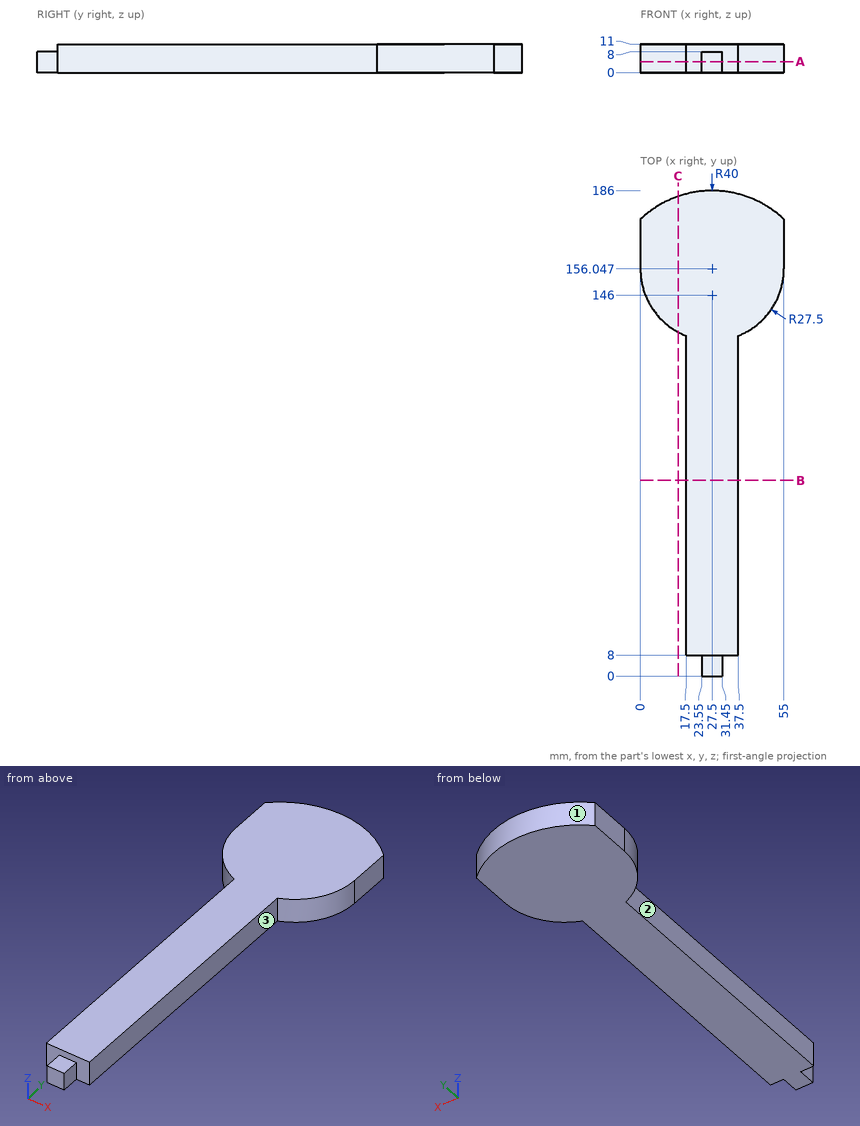
Input: dimensioned drawing with shaded views. Units: mm. Origin: part minimum x, y, z. A direction names the side the tool comes from. Give positions to 0.01 mm unless a question says otherwise; leave off trailing zeros. Loops run counter-clockwise (first coordinate to the right, second up) from the corner with the lowest first, then second, coordinate; pieces in that order, holes last. Notation, with made-up numbers: M -12.75,1 L 29.25,1 A12 ccw 29.25,10 Z; hole C 33,25.5 d2. An arc over 180 degrees is marked long. Put each result on its own line as item: value. Start each with the question number.
1) Access query for the marked faces 1, 2 and 3. Directions: +Z, -Z, +X, -X, +Y, -Y. A direction counts if a zero-diameter tool reaches every point of the face in a straight line with its end or side. Return the directions, or none.
2) Ray query, line 1 along X through (y, z) = (45.5, 10.75); line 2 along Y through (x, z) = (27, 2.75); line 3 along Y through (x, z) = (40, 6.75). Return the intervals inside material, ascending.
3) Cut plane A-A (z = 4.25). Output: boundary loops of the cut face in (x, y), then the cut area to 3 significant figures.
4) Contact query for flat-ended pins moving along their axis: pin 1 (2 mm diameter, centred on y = 54.5, z = 5, fed in from -X); pin 2 (2 mm diameter, centred on x = 10, z = 5.5, fed in from -Y); pin 3 (2 mm diameter, centred on x = 40, z = 3, fed in from -Y). Output: stop coordinate, or through.
5) Cut plane C-C (x = 14.5). Output: boundary loops of the cut face in (y, z) (1 decimal), then the cut area to 3 significant figures.
6) Cut plane B-B (y = 75). Output: boundary loops of the cut face in (x, z).
Verdict:
1. face 1: +Z, -Z, +Y
1. face 2: +Z, -Z, -X, -Y
1. face 3: +Z, -Z, +X, -Y
2. line 1: 17.5 to 37.5
2. line 2: 0 to 186
2. line 3: 131.55 to 184
3. outline: M 0,156.05 A27.5 ccw 17.5,130.43 L 17.5,8 L 23.55,8 L 23.55,0 L 31.45,0 L 31.45,8 L 37.5,8 L 37.5,130.43 A27.5 ccw 55,156.05 L 55,175.05 A40 ccw 0,175.05 Z
3. area: 5,130 mm2
4. pin 1: x = 17.5
4. pin 2: y = 134.05
4. pin 3: y = 131.07
5. outline: M 131.8,0 L 183.8,0 L 183.8,11 L 131.8,11 Z
5. area: 572 mm2
6. outline: M 17.5,0 L 37.5,0 L 37.5,11 L 17.5,11 Z
